Design review of the part built by this model. Coordinates are the model's own, in mm. Face numbers are marked on the shaded views. A direction names the side the tool comes from. Round coordinates to 2 decimals unless told otherwise and drop trailing zeros. Order: outer loops, then holes, each group sorted by start corner. A loop starts at its lowest first (then second) coordinate and runs counter-clockwise, first axis right, second up.
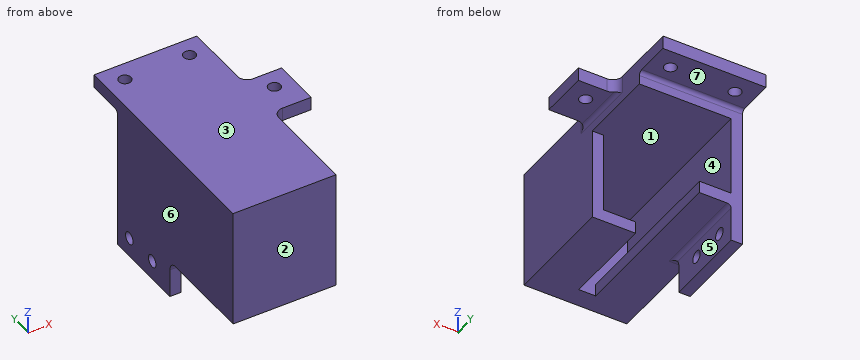
from build123d import *

# Parameters (mm, degrees)
BOSS_EXTRUDE1_DEPTH      = 48
SKETCH2_W                = 53.78
SKETCH2_H                = 62.166
BOSS_EXTRUDE2_DEPTH      = 10
BOSS_EXTRUDE3_DEPTH      = 40
BOSS_EXTRUDE3_DEPTH_BACK = 4.425
SKETCH6_W                = 20
SKETCH6_H                = 19.425
CUT_EXTRUDE3_DEPTH       = 125.870331368
SKETCH7_W                = 53.78
SKETCH7_H                = 7
BOSS_EXTRUDE4_DEPTH      = 20
SKETCH9_W                = 16.61
SKETCH9_H                = 6.39
BOSS_EXTRUDE5_DEPTH      = 40
SKETCH4_R                = 3.175
CUT_EXTRUDE1_DEPTH       = 137.084033597
SKETCH5_R                = 3.175
CUT_EXTRUDE2_DEPTH       = 140.687507158
SKETCH8_R                = 3.175
CUT_EXTRUDE4_DEPTH       = 140.687507158
FILLET1_R                = 2
FILLET2_R                = 5


with BuildPart() as part:
    # Sketch1 → Boss-Extrude1 (new body)
    with BuildSketch(Plane(origin=(0, 0, 0), x_dir=(1, 0, 0), z_dir=(0, 1, 0))):
        Polygon((4.39, 21), (4.39, 27.39), (26.89, 27.39), (26.89, -34.776), (-26.89, -34.776), (-26.89, 27.39), (-4.39, 27.39), (-4.39, 21), (-21, 21), (-21, -21), (21, -21), (21, 21), align=None)
    extrude(amount=BOSS_EXTRUDE1_DEPTH)

    # Sketch2 → Boss-Extrude2 (add)
    with BuildSketch(Plane(origin=(0, 0, 0), x_dir=(1, 0, 0), z_dir=(0, 1, 0))):
        with Locations((0, -3.693)):
            Rectangle(SKETCH2_W, SKETCH2_H)
    extrude(amount=-BOSS_EXTRUDE2_DEPTH)

    # Sketch3 → Boss-Extrude3 (add, two sides: drawn at the far end of the back side and taken through both)
    with BuildSketch(Plane(origin=(0, 48, 0), x_dir=(1, 0, 0), z_dir=(0, 1, 0)).offset(-BOSS_EXTRUDE3_DEPTH_BACK)):
        Polygon((26.89, -21), (26.89, -27.776), (46.89, -27.776), (46.89, -34.776), (-26.89, -34.776), (-26.89, 47.39), (-21, 47.39), (-21, -21), align=None)
    extrude(amount=BOSS_EXTRUDE3_DEPTH + BOSS_EXTRUDE3_DEPTH_BACK)

    # Sketch6 → Cut-Extrude3 (cut, through all)
    with BuildSketch(Plane(origin=(0, 0, 27.776), x_dir=(-1, 0, 0), z_dir=(0, 0, -1))):
        with Locations((-36.89, 78.2875)):
            Rectangle(SKETCH6_W, SKETCH6_H)
    extrude(amount=-CUT_EXTRUDE3_DEPTH, mode=Mode.SUBTRACT)

    # Sketch7 → Boss-Extrude4 (add)
    with BuildSketch(Plane(origin=(0, 88, 0), x_dir=(1, 0, 0), z_dir=(0, 1, 0))):
        with Locations((0, -31.276)):
            Rectangle(SKETCH7_W, SKETCH7_H)
    extrude(amount=BOSS_EXTRUDE4_DEPTH)

    # Sketch9 → Boss-Extrude5 (add)
    with BuildSketch(Plane(origin=(0, 48, 0), x_dir=(1, 0, 0), z_dir=(0, 1, 0))):
        with Locations((-12.695, 24.195)):
            Rectangle(SKETCH9_W, SKETCH9_H)
    extrude(amount=BOSS_EXTRUDE5_DEPTH)

    # Sketch4 → Cut-Extrude1 (cut, through all)
    with BuildSketch(Plane(origin=(-21, 0, 0), x_dir=(0, 0, -1), z_dir=(1, 0, 0))):
        with Locations((37.39, 78)):
            Circle(SKETCH4_R)
        with Locations((37.39, 58.575)):
            Circle(SKETCH4_R)
    extrude(amount=-CUT_EXTRUDE1_DEPTH, mode=Mode.SUBTRACT)

    # Sketch5 → Cut-Extrude2 (cut, through all)
    with BuildSketch(Plane.XY.offset(27.776)):
        with Locations((36.89, 58.575)):
            Circle(SKETCH5_R)
    extrude(amount=CUT_EXTRUDE2_DEPTH, mode=Mode.SUBTRACT)

    # Sketch8 → Cut-Extrude4 (cut, through all)
    with BuildSketch(Plane(origin=(0, 0, 27.776), x_dir=(-1, 0, 0), z_dir=(0, 0, -1))):
        with Locations((-16.89, 98)):
            Circle(SKETCH8_R)
        with Locations((16.89, 98)):
            Circle(SKETCH8_R)
    extrude(amount=-CUT_EXTRUDE4_DEPTH, mode=Mode.SUBTRACT)

    # Fillet1
    fillet1_edges = [part.edges().sort_by_distance(p)[0] for p in [
        (26.89, 56.075, 27.776),
        (0, 88, 27.776),
        (-21, 65.7875, -27.39),
    ]]
    fillet(fillet1_edges, radius=FILLET1_R)

    # Fillet2
    fillet2_edges = [part.edges().sort_by_distance(p)[0] for p in [
        (-22.945, 43.575, -27.39),
    ]]
    fillet(fillet2_edges, radius=FILLET2_R)
    fillet2_2_edges = [part.edges().sort_by_distance(p)[0] for p in [
        (26.89, 68.575, 30.276),
    ]]
    fillet(fillet2_2_edges, radius=FILLET2_R)
    fillet2_3_edges = [part.edges().sort_by_distance(p)[0] for p in [
        (26.89, 43.575, 30.276),
    ]]
    fillet(fillet2_3_edges, radius=FILLET2_R)


solid = part.part
1) Take a section at C-C on z = -38. Give the boundary of the cut face in (x, y) (3 decimals), plus the area to 3 significant figures.
Results:
outline: (-26.89, 43.575) - (-21, 43.575) - (-21, 55.459) - (-26.89, 55.459) - close; (-26.89, 61.691) - (-21, 61.691) - (-21, 74.884) - (-26.89, 74.884) - close; (-26.89, 81.116) - (-21, 81.116) - (-21, 88) - (-26.89, 88) - close
area: 188 mm2
2) To check wall thickness, follow line 1 along Z through (x, y) = (-16.5, 85); line 2 along Y through (x, z) = (16.89, 31.5) (3 decimals); line 3 along X through (y, z) = (10, 15). State the ranges of each line that lie inside material, in increasing order.
Results:
line 1: z = -27.39 to -21, 21 to 34.78
line 2: y = -10 to 94.825, 101.175 to 108
line 3: x = -26.89 to -21, 21 to 26.89
3) Take a section at D-D on x = -3. Give the boundary of the cut face in (y, z).
Results:
outline: (-10, -27.39) - (0, -27.39) - (0, 21) - (88, 21) - (88, 25.78) arc R2 cw to (90, 27.78) - (108, 27.78) - (108, 34.78) - (-10, 34.78) - close
4) The part is to be moulded in two halves that separate along Z. For the marked faces 1, 2, 3 and 4, say which applies: released by +Z, released by -Z, zero draft, split by the parting line, or undercut.
Results:
face 1: undercut
face 2: zero draft
face 3: released by +Z
face 4: undercut
5) For the marked faces 5, 6 and 7, list the 3-axis set-ups (+Z, -Z, +X, -X, +Y, -Y) from which the entire face can be reached by the end or side of a thin tool; tool diameter is ignored.
Results:
face 5: -Z, +X, +Y, -Y
face 6: +Z, -Z, -X, +Y, -Y
face 7: -Z, +X, -X, +Y
6) Take a section at B-B on y = 78. Give the boundary of the cut face in (x, z) (3 decimals).
Results:
outline: (-26.89, -47.39) - (-21, -47.39) - (-21, -40.565) - (-26.89, -40.565) - close; (-26.89, -34.215) - (-21, -34.215) - (-21, -29.39) arc R2 cw to (-19, -27.39) - (-4.39, -27.39) - (-4.39, -21) - (-21, -21) - (-21, 21) - (26.89, 21) - (26.89, 34.776) - (-26.89, 34.776) - close
7) Clearance check with flat-ended pins moving along their axes: P1, Ø14.5, axis at x = 13.5, y = 26.5, coming from the -Z side; P2, Ø8, axis at x = 29, y = 72.5, coming from the -Z side; P3, Ø1, axis at x = -1, z = -19.5, coming from the +Y side. State where each tip first meets the part, or that it passes through.
Results:
P1: stops at z = -27.39
P2: stops at z = 21
P3: stops at y = 0
8) Take a section at A-A on x = -16.89. Give the boundary of the cut face in (y, z) (3 decimals).
Results:
outline: (-10, -27.39) - (88, -27.39) - (88, -21) - (0, -21) - (0, 21) - (88, 21) - (88, 25.776) arc R2 cw to (90, 27.776) - (94.825, 27.776) - (94.825, 34.776) - (-10, 34.776) - close; (101.175, 27.776) - (108, 27.776) - (108, 34.776) - (101.175, 34.776) - close
